Could you check a few things on this model? Use its own coordinates, in mm. Face numbers are marked on the shaded views. A direction names the side the tool comes from. Round coordinates to 2 decimals unless told otherwise and drop trailing zeros. Loops run counter-clockwise (first coordinate to the right, second up) from the corner with the lowest first, then second, coordinate; pieces in that order, holes last. Notation, with made-up numbers: (-14, -9.5) -> (20, -9.5) arc R8 ccw to (20, -4.5) -> close; hole circle Ø8 at (-25.75, -10). An arc over 180 degrees is marked (long way). Put each result on its own line as item: value. Start each with the question number.
1. Imagine slicing it at B-B, the plane y = -11.5. Count the separate pieces of the cut face and the enclosed holes in it, and give its area (3 significant figures).
2. I need wall thicknesses on line 1 (Z direction, x = -37.5, y = 4.9); line 2 (X direction, y = 7.1, z = -24); line 3 (Y direction, x = 29, z = 0). Which ranges of each line are inside material? Lowest first, please. Write a range as [from, to].
3. If we mould it in two halves opening along X, with no side actions, what happens to the marked faces 1, 2, 3 and 4? For each: pulls with the +X half, pulls with the -X half, needs draft (parallel to the pull), parting line crosses it, or undercut.
4. I'm going to push flat-ended pins straight in: P1, Ø4, axis at y = -39.5, z = -7, coming from the +X side (3 decimals); P2, Ø3, axis at x = -30, y = -11.5, coming from the +Z side; P3, Ø8, axis at x = 30, z = -6, coming from the -Y side. Where does each tip first touch, or does it pass through?
5. Imagine slicing it at A-A, the plane z = 7. Please give me the cut outline in (x, y) (3 decimals), and give its area (3 significant figures).
6. Imagine slicing it at C-C, the plane x = -22. Please give me the cut outline in (y, z), and give its area (3 significant figures).
7. Which directions (+Z, -Z, +X, -X, +Y, -Y) give clear straight access to the entire face, cutting with the end or side of a thin tool? Please do the marked faces 5 and 6.
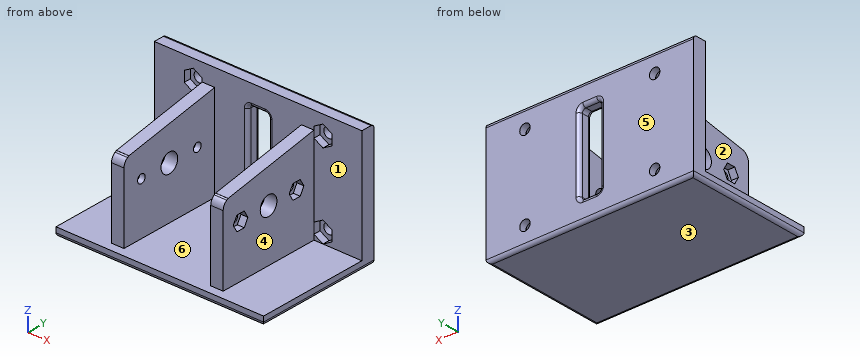
```python
from build123d import *
from OCP.BRepFilletAPI import BRepFilletAPI_MakeChamfer

# Parameters (mm, degrees)
SKETCH1_W               = 120
SKETCH1_H               = 70
SKETCH1_R               = 3
SKETCH1_W_2             = 12
SKETCH1_H_2             = 46
BOSS_EXTRUDE1_DEPTH     = 8
FILLET1_R               = 2
SKETCH2_W               = 120
SKETCH2_H               = 5
BOSS_EXTRUDE2_DEPTH     = 65
SKETCH3_W               = 7.2
SKETCH3_H               = 60
BOSS_EXTRUDE3_DEPTH     = 45
CUT_EXTRUDE1_DEPTH      = 119.172228654
CUT_EXTRUDE1_DEPTH_BACK = 119.172228654
SKETCH4_R               = 5.5
SKETCH4_R_2             = 2.5
CUT_EXTRUDE2_DEPTH      = 4
CUT_EXTRUDE3_DEPTH      = 4
CUT_EXTRUDE4_DEPTH      = 4
CHAMFER1_SIZE           = 10
CHAMFER1_SIZE2          = 56.712818196
FILLET3_R               = 2
CHAMFER2_SIZE           = 2
CHAMFER2_SIZE2          = 3.200669058
FILLET4_R               = 5


with BuildPart() as part:
    # Sketch1 → Boss-Extrude1 (new body)
    with BuildSketch(Plane(origin=(0, 0, 0), x_dir=(1, 0, 0), z_dir=(0, 1, 0))):
        Rectangle(SKETCH1_W, SKETCH1_H)
        with Locations(Location((-37.5, 24, 0), (0, 0, 270))):
            Circle(SKETCH1_R, mode=Mode.SUBTRACT)
        with Locations(Location((-37.5, -24, 0), (0, 0, 90))):
            Circle(SKETCH1_R, mode=Mode.SUBTRACT)
        with Locations(Location((37.5, 24, 0), (0, 0, 90))):
            Circle(SKETCH1_R, mode=Mode.SUBTRACT)
        with Locations(Location((37.5, -24, 0), (0, 0, 270))):
            Circle(SKETCH1_R, mode=Mode.SUBTRACT)
        Rectangle(SKETCH1_W_2, SKETCH1_H_2, mode=Mode.SUBTRACT)
    extrude(amount=BOSS_EXTRUDE1_DEPTH)

    # Fillet1
    fillet1_edges = [part.edges().sort_by_distance(p)[0] for p in [
        (-6, 4, -23),
        (-6, 4, 23),
        (6, 4, 23),
        (6, 4, -23),
    ]]
    fillet(fillet1_edges, radius=FILLET1_R)

    # Sketch2 → Boss-Extrude2 (add)
    with BuildSketch(Plane.XZ):
        with Locations((0, -32.5)):
            Rectangle(SKETCH2_W, SKETCH2_H)
    extrude(amount=BOSS_EXTRUDE2_DEPTH)

    # Sketch3 → Boss-Extrude3 (add)
    with BuildSketch(Plane.XY.offset(-30)):
        with Locations((-28.675, -30)):
            Rectangle(SKETCH3_W, SKETCH3_H)
        with Locations((28.675, -30)):
            Rectangle(SKETCH3_W, SKETCH3_H)
    extrude(amount=BOSS_EXTRUDE3_DEPTH)

    # Sketch4 → Cut-Extrude1 (cut, two sides: drawn at the far end of the back side and taken through both)
    with BuildSketch(Plane.ZY.offset(32.275).offset(-CUT_EXTRUDE1_DEPTH_BACK)):
        with Locations((0, -30)):
            Circle(SKETCH4_R)
        with Locations((0, -11.5)):
            Circle(SKETCH4_R_2)
        with Locations((0, -48.5)):
            Circle(SKETCH4_R_2)
    extrude(amount=CUT_EXTRUDE1_DEPTH + CUT_EXTRUDE1_DEPTH_BACK, mode=Mode.SUBTRACT)

    # Sketch5 → Cut-Extrude2 (cut)
    with BuildSketch(Plane.ZY.offset(32.275)):
        Polygon((4.2, -9.075128869), (0, -6.650257739), (-4.2, -9.075128869), (-4.2, -13.924871131), (0, -16.349742261), (4.2, -13.924871131), align=None)
        Polygon((4.2, -46.075128869), (0, -43.650257739), (-4.2, -46.075128869), (-4.2, -50.924871131), (0, -53.349742261), (4.2, -50.924871131), align=None)
    extrude(amount=-CUT_EXTRUDE2_DEPTH, mode=Mode.SUBTRACT)

    # Sketch6 → Cut-Extrude3 (cut)
    with BuildSketch(Plane(origin=(32.275, 0, 0), x_dir=(0, 0, -1), z_dir=(1, 0, 0))):
        Polygon((4.2, -13.924871131), (4.2, -9.075128869), (0, -6.650257739), (-4.2, -9.075128869), (-4.2, -13.924871131), (0, -16.349742261), align=None)
        Polygon((-4.2, -46.075128869), (-4.2, -50.924871131), (0, -53.349742261), (4.2, -50.924871131), (4.2, -46.075128869), (0, -43.650257739), align=None)
    extrude(amount=-CUT_EXTRUDE3_DEPTH, mode=Mode.SUBTRACT)

    # Sketch7 → Cut-Extrude4 (cut)
    with BuildSketch(Plane.XZ):
        Polygon((42.7, -20.9977786), (37.5, -17.9955572), (32.3, -20.9977786), (32.3, -27.0022214), (37.5, -30.0044428), (42.7, -27.0022214), align=None)
        Polygon((42.7, 27.0022214), (37.5, 30.0044428), (32.3, 27.0022214), (32.3, 20.9977786), (37.5, 17.9955572), (42.7, 20.9977786), align=None)
        Polygon((-42.7, -27.0022214), (-42.7, -20.9977786), (-37.5, -17.9955572), (-32.3, -20.9977786), (-32.3, -27.0022214), (-37.5, -30.0044428), align=None)
        Polygon((-42.7, 20.9977786), (-42.7, 27.0022214), (-37.5, 30.0044428), (-32.3, 27.0022214), (-32.3, 20.9977786), (-37.5, 17.9955572), align=None)
    extrude(amount=-CUT_EXTRUDE4_DEPTH, mode=Mode.SUBTRACT)

    # Chamfer1
    chamfer1_edges = [part.edges().sort_by_distance(p)[0] for p in [
        (28.675, 0, 15),
        (-28.675, 0, 15),
    ]]
    chamfer1_side = [part.faces().sort_by_distance(p)[0] for p in [
        (-58.635265594, 0, 2.5),
    ]]
    chamfer(chamfer1_edges, length=CHAMFER1_SIZE, length2=CHAMFER1_SIZE2, reference=chamfer1_side[0])

    # Fillet3
    fillet3_edges = [part.edges().sort_by_distance(p)[0] for p in [
        (0, 8, 35),
        (0, 0, 23),
        (0, 8, 23),
        (6, 0, 0),
        (6, 8, 0),
        (-6, 0, 0),
        (-6, 8, 0),
        (0, 0, -23),
        (0, 8, -23),
        (5.414213562, 0, 22.414213562),
        (5.414213562, 8, 22.414213562),
        (-5.414213562, 0, 22.414213562),
        (-5.414213562, 8, 22.414213562),
        (5.414213562, 0, -22.414213562),
        (5.414213562, 8, -22.414213562),
        (-5.414213562, 0, -22.414213562),
        (-5.414213562, 8, -22.414213562),
        (0, -65, -35),
        (-60, -28.5, -35),
        (60, -28.5, -35),
        (0, 8, -35),
    ]]
    fillet(fillet3_edges, radius=FILLET3_R)

    # Chamfer2: one chamfer whose edges measure the first distance from different faces: ONE call of the kernel's chamfer builder (chamfer() names one face for all edges)
    chamfer2_edges_1 = [part.edges().sort_by_distance(p)[0] for p in [
        (28.675, -60, 15),
    ]]
    chamfer2_side_1 = [part.faces().sort_by_distance(p)[0] for p in [
        (28.675, -60, -7.5),
    ]]
    chamfer2_edges_2 = [part.edges().sort_by_distance(p)[0] for p in [
        (-28.675, -60, 15),
    ]]
    chamfer2_side_2 = [part.faces().sort_by_distance(p)[0] for p in [
        (-28.675, -60, -7.5),
    ]]
    chamfer2 = BRepFilletAPI_MakeChamfer(part.part.solid().wrapped)
    for e in chamfer2_edges_1:
        chamfer2.Add(CHAMFER2_SIZE, CHAMFER2_SIZE2, e.wrapped, chamfer2_side_1[0].wrapped)  # the first distance lies on this face
    for e in chamfer2_edges_2:
        chamfer2.Add(CHAMFER2_SIZE, CHAMFER2_SIZE2, e.wrapped, chamfer2_side_2[0].wrapped)  # the first distance lies on this face
    add(Compound.cast(chamfer2.Shape()), mode=Mode.REPLACE)

    # Fillet4
    fillet4_edges = [part.edges().sort_by_distance(p)[0] for p in [
        (28.675, -60, 13),
        (-28.675, -60, 13),
    ]]
    fillet(fillet4_edges, radius=FILLET4_R)


solid = part.part
```
Entries:
1. separate pieces: 3
1. enclosed holes: 0
1. area: 1,260 mm^2
2. line 1: [-35, -27], [-21, 21], [27, 35]
2. line 2: [-60, -40.5], [-34.5, 34.5], [40.5, 60]
2. line 3: [-60, -53.35], [-43.65, -35.5], [-24.5, -16.35], [-6.65, 8]
3. face 1: undercut
3. face 2: pulls with the -X half
3. face 3: needs draft
3. face 4: pulls with the +X half
4. P1: x = 32.275
4. P2: z = 23.24
4. P3: y = -60
5. outline: (-60, 0) -> (-32.275, 0) -> (-32.275, -60) -> (-25.075, -60) -> (-25.075, 0) -> (-8, 0) arc R2 ccw to (-6, 2) -> (-6, 6) arc R2 ccw to (-8, 8) -> (-60, 8) -> close; (6, 2) arc R2 ccw to (8, 0) -> (25.075, 0) -> (25.075, -60) -> (32.275, -60) -> (32.275, 0) -> (60, 0) -> (60, 8) -> (8, 8) arc R2 ccw to (6, 6) -> close
5. area: 1,720 mm^2
6. outline: (-65, -33) arc R2 ccw to (-63, -35) -> (6, -35) arc R2 ccw to (8, -33) -> (8, 33) arc R2 ccw to (6, 35) -> (0, 35) -> (0, -30) -> (-65, -30) -> close
6. area: 882 mm^2
7. face 5: +Z, -Z, +X, -X, +Y
7. face 6: +Z, -Y
